Read the model definition and answer for the solid it produces. Units are mm, in the model's axes. Face numbers are marked on the shaded views. A direction names the side the tool comes from. Coordinates: 2 decimals unless noted, no trailing zeros. Write each loop counter-clockwise with the first axis right and the second up, starting at its lowest first coordinate (ties: lowest second). Pieces come first, ordered by that corner, then holes. Notation, with made-up numbers: M 84.25,-10.5 L 133.25,-10.5 A26 ccw 133.25,4.5 Z; hole C -15,76.5 d3. An arc over 180 degrees is marked long. Write item = value, one per line.
from build123d import *

# Parameters (mm, degrees)
F2_SIZE = 0.396875


# Not quite as in the source:
# - a feature names something its author has since deleted; it is built from what else it names


with BuildPart() as f1:
    # F0 (on Front) → F1 (revolve)
    with BuildSketch(Plane.XZ):
        with BuildLine():
            Line((0, 8.1915), (0, 12.7))
            Line((0, 12.7), (-5.715, 12.7))
            Line((-5.715, 12.7), (-24.0689650903, 6.35))
            ThreePointArc((-24.0689650903, 6.35), (-26.8959476355, 3.7184476355), (-27.94, 0))
            Line((-27.94, 0), (22.225, 0))
            Line((22.225, 0), (22.225, 5.334))
            Line((22.225, 5.334), (19.05, 5.334))
            Line((19.05, 5.334), (19.05, 4.1656))
            Line((19.05, 4.1656), (14.605, 4.1656))
            Line((14.605, 4.1656), (14.605, 5.334))
            Line((14.605, 5.334), (10.16, 5.334))
            Line((10.16, 5.334), (8.89, 6.604))
            Line((8.89, 6.604), (1.5875, 6.604))
            ThreePointArc((1.5875, 6.604), (0.4649679849, 7.0689679849), (0, 8.1915))
        make_face()
    revolve(axis=Axis((-2.8575, 0, 0), (-1, 0, 0)))

    # F2
    f2_edges = [f1.edges().sort_by_distance(p)[0] for p in [
        (0, 0, -12.7),
    ]]
    chamfer(f2_edges, length=F2_SIZE)


solid = f1.part
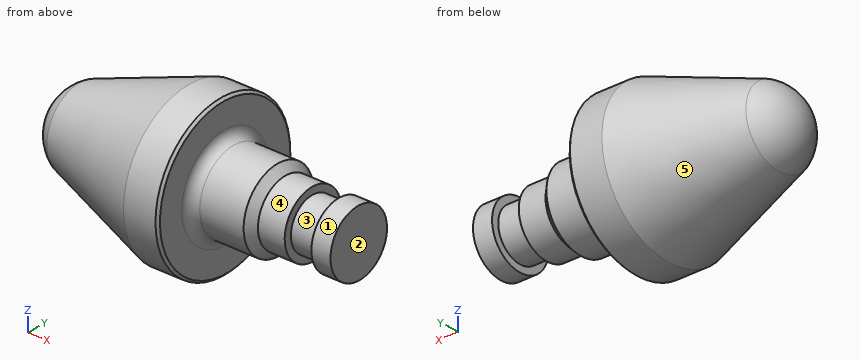
Item 1: Which of the six approach directions +Z, -Z, +X, -X, +Y, -Y give full straight-line access (tool end or side, diameter ignored) to the marked faces 4 and 5?
Worked answers:
face_4 = +X
face_5 = -X
Item 2: Consider line 1 along X through (y, z) = (-3.5, -3.25) (3 decimals); line 2 along X through (y, z) = (-5.75, 7); line 3 along Z through (x, y) = (0.5, 2). Determine where each line is inside the solid, lowest interval first. Write a range as from..to.
Worked answers:
line_1 = -26.109..14.605, 19.05..22.225
line_2 = -16.24..0
line_3 = -6.74..6.74
Item 3: Find section C-C (x = 13.5). Determine the outline of the cut face in (y, z), and give its area (3 significant figures).
Worked answers:
outline = C 0,0 d10.67
area = 89.4 mm²
Item 4: Find section D-D (x = -3). Determine the outline of the cut face in (y, z), and give its area (3 significant figures).
Worked answers:
outline = C 0,0 d25.4
area = 507 mm²
Item 5: For a pull along X with two mould halves and no side action, classify the marked faces 1, 2 and 3 as released by +X, released by -X, zero draft, split by the parting line, or undercut.
Worked answers:
face_1 = zero draft
face_2 = released by +X
face_3 = undercut
Item 6: Flat-ended cylindrical pins translate along their axes: pin 1 (5.5 mm diameter, centred on y = 1, z = -2, fed in from -X); pin 2 (2 mm diameter, centred on x = -8, z = 7, fed in from -Y); pin 3 (5 mm diameter, centred on x = -15, y = -4, fed in from +Z); pin 4 (1.5 mm diameter, centred on y = 8, z = -8.5, fed in from +X). Find the tip coordinate at first contact, or state that the pin passes through.
Worked answers:
pin_1 = -27.94
pin_2 = -10.41
pin_3 = 9.87
pin_4 = 0
